Could you check a few things on this model? Use its own coordinates, in mm. A direction names the side the tool comes from. Give positions to 0.01 mm unless a question says otherwise; leave off trailing zeros. Loops run counter-clockwise (first coordinate to the right, second up) from the corner with the lowest first, then second, coordinate; pieces in that order, holes last. Notation, with made-up numbers: M -36,45 L 9,45 A14 ccw 9,50 Z; hole C -38,79.5 d11. An arc over 180 degrees is marked long. Use a Markdown table: item, result. Add a question column.
1) Suppose I cut it at B-B on y = 22. Count the separate pieces of the cut face and the enclosed holes in it, and give its area (3 significant figures).
2) If I drill on line 1 along X through (y, z) = (8.5, 23.75); line 2 along X through (y, z) = (16.5, 12); line 3 along Y through (x, z) = (-50.5, 4.5), over which ranges is the centre line in solid material (lowest first)? Write a range as [from, to].
3) Suppose I cut it at A-A on x = -41. List the corners of the cut face in (y, z) for me, and give its area (3 significant figures).
4) We'd pull the mould along X, two halves only. Please class faces 1 (the flat face through (-1, 1, 0)), 2 (the flat face through (-38, 0, 13)), 3 (the flat face through (-76.2, -1, 13)): +X half, -X half, draft (parallel to the pull), parting line (faces both ways), or undercut.
5) Which directions (+Z, -Z, +X, -X, +Y, -Y) give clear straight access to the entire face, cutting with the end or side of a thin tool? Please do faces 4 (the flat face through (76.2, -1, 13)), 5 (the flat face through (-38, 25.4, 13)).
```python
from build123d import *

# Parameters (mm, degrees)
F0_W     = 152.4
F0_H     = 101.6
F1_DEPTH = 25.4
F2_W     = 25.4
F2_H     = 25.4
F3_DEPTH = 25.401
F4_W     = 25.4
F4_H     = 25.4
F5_DEPTH = 25.401
F5_TAPER = -5


with BuildPart() as f1:
    # F0 (on Top) → F1 (new body)
    with BuildSketch(Plane.XY):
        Rectangle(F0_W, F0_H)
    extrude(amount=F1_DEPTH)

    # F2 (on face) → F3 (cut, through all)
    with BuildSketch(Plane.XY.offset(25.4)):
        with Locations((-38.1, 12.7)):
            Rectangle(F2_W, F2_H)
    extrude(amount=-F3_DEPTH, mode=Mode.SUBTRACT)

    # F4 (on face) → F5 (cut, through all)
    with BuildSketch(Plane.XY.offset(25.4)):
        with Locations((38.1, 14.9531663823)):
            Rectangle(F4_W, F4_H)
    extrude(amount=-F5_DEPTH, taper=F5_TAPER, mode=Mode.SUBTRACT)


solid = f1.part
```
Answer block:
| question | item | result |
|---|---|---|
| 1 | separate pieces | 3 |
| 1 | enclosed holes | 0 |
| 1 | area | 2,520 mm^2 |
| 2 | line 1 | x = [-76.2, -50.8], [-25.4, 25.26], [50.94, 76.2] |
| 2 | line 2 | x = [-76.2, -50.8], [-25.4, 24.23], [51.97, 76.2] |
| 2 | line 3 | y = [-50.8, 0], [25.4, 50.8] |
| 3 | outline | M -50.8,0 L 0,0 L 0,25.4 L -50.8,25.4 Z; M 25.4,0 L 50.8,0 L 50.8,25.4 L 25.4,25.4 Z |
| 3 | area | 1,940 mm^2 |
| 4 | face 1 | draft |
| 4 | face 2 | undercut |
| 4 | face 3 | -X half |
| 5 | face 4 | +Z, -Z, +X, +Y, -Y |
| 5 | face 5 | +Z, -Z |
